```python
from build123d import *

# Parameters (mm, degrees)
BOSS_EXTRUDE1_DEPTH = 513.461
SKETCH2_R           = 19.05
CUT_EXTRUDE1_DEPTH  = 31.75
SKETCH3_R           = 3.2258
CUT_EXTRUDE2_DEPTH  = 31.75
SKETCH4_R           = 11.500000003
CUT_EXTRUDE3_DEPTH  = 499.872


with BuildPart() as part:
    # Sketch1 → Boss-Extrude1 (new body)
    with BuildSketch(Plane.XY):
        with BuildLine():
            Line((-159.385, 0), (-158.115, 0))
            ThreePointArc((-158.115, 0), (-154.073884746, -1.673884746), (-152.4, -5.715))
            Line((-152.4, -5.715), (-152.4, -16.91))
            ThreePointArc((-152.4, -16.91), (-150.726115254, -20.951115254), (-146.685, -22.625))
            Line((-146.685, -22.625), (-125.96, -22.625))
            ThreePointArc((-125.96, -22.625), (-121.918884746, -24.298884746), (-120.245, -28.34))
            Line((-120.245, -28.34), (-120.245, -57.40750012))
            ThreePointArc((-120.245, -57.40750012), (-118.571115254, -61.448615374), (-114.53, -63.12250012))
            Line((-114.53, -63.12250012), (-107.315, -63.12250012))
            ThreePointArc((-107.315, -63.12250012), (-103.273884746, -61.448615374), (-101.6, -57.40750012))
            Line((-101.6, -57.40750012), (-101.6, 0))
            Line((-101.6, 0), (-101.6, 38.17350945))
            ThreePointArc((-101.6, 38.17350945), (-99.926115254, 42.214624704), (-95.885, 43.88850945))
            Line((-95.885, 43.88850945), (95.885, 43.88850945))
            ThreePointArc((95.885, 43.88850945), (99.926115254, 42.214624704), (101.6, 38.17350945))
            Line((101.6, 38.17350945), (101.6, 0))
            Line((101.6, 0), (101.6, -57.40750012))
            ThreePointArc((101.6, -57.40750012), (103.273884746, -61.448615374), (107.315, -63.12250012))
            Line((107.315, -63.12250012), (114.53, -63.12250012))
            ThreePointArc((114.53, -63.12250012), (118.571115254, -61.448615374), (120.245, -57.40750012))
            Line((120.245, -57.40750012), (120.245, -28.34))
            ThreePointArc((120.245, -28.34), (121.918884746, -24.298884746), (125.96, -22.625))
            Line((125.96, -22.625), (146.685, -22.625))
            ThreePointArc((146.685, -22.625), (150.726115254, -20.951115254), (152.4, -16.91))
            Line((152.4, -16.91), (152.4, -5.715))
            ThreePointArc((152.4, -5.715), (154.073884746, -1.673884746), (158.115, 0))
            Line((158.115, 0), (159.385, 0))
            ThreePointArc((159.385, 0), (163.426115254, 1.673884746), (165.1, 5.715))
            Line((165.1, 5.715), (165.1, 59.52))
            ThreePointArc((165.1, 59.52), (157.660512242, 77.480512242), (139.7, 84.92))
            Line((139.7, 84.92), (-139.7, 84.92))
            ThreePointArc((-139.7, 84.92), (-157.660512242, 77.480512242), (-165.1, 59.52))
            Line((-165.1, 59.52), (-165.1, 5.715))
            ThreePointArc((-165.1, 5.715), (-163.426115254, 1.673884746), (-159.385, 0))
        make_face()
    extrude(amount=BOSS_EXTRUDE1_DEPTH)

    # Sketch2 → Cut-Extrude1 (cut)
    with BuildSketch(Plane(origin=(0, 84.92, 0), x_dir=(1, 0, 0), z_dir=(0, 1, 0))):
        with Locations(Location((-50.8, -25.4, 0), (0, 0, 270))):
            Circle(SKETCH2_R)
        with Locations(Location((50.8, -25.4, 0), (0, 0, 270))):
            Circle(SKETCH2_R)
        with Locations(Location((50.8, -488.061, 0), (0, 0, 270))):
            Circle(SKETCH2_R)
        with Locations(Location((-50.8, -488.061, 0), (0, 0, 270))):
            Circle(SKETCH2_R)
    extrude(amount=-CUT_EXTRUDE1_DEPTH, mode=Mode.SUBTRACT)

    # Sketch3 → Cut-Extrude2 (cut)
    with BuildSketch(Plane(origin=(0, 53.17, 0), x_dir=(1, 0, 0), z_dir=(0, 1, 0))):
        with Locations(Location((-50.8, -25.4, 0), (0, 0, 270))):
            Circle(SKETCH3_R)
        with Locations(Location((50.8, -25.4, 0), (0, 0, 270))):
            Circle(SKETCH3_R)
        with Locations(Location((50.8, -488.061, 0), (0, 0, 270))):
            Circle(SKETCH3_R)
        with Locations(Location((-50.8, -488.061, 0), (0, 0, 270))):
            Circle(SKETCH3_R)
    extrude(amount=-CUT_EXTRUDE2_DEPTH, mode=Mode.SUBTRACT)

    # Sketch4 → Cut-Extrude3 (cut)
    with BuildSketch(Plane.ZY.offset(165.1)):
        with Locations(Location((344.866041788, 12.13850945, 0), (0, 0, 326.043312317))):
            Circle(SKETCH4_R)
        with Locations(Location((197.228541788, 12.13850945, 0), (0, 0, 326.043312317))):
            Circle(SKETCH4_R)
    extrude(amount=-CUT_EXTRUDE3_DEPTH, mode=Mode.SUBTRACT)


solid = part.part
```
Could you check a few things on this model? Use its own coordinates, in mm. A direction names the side the tool comes from. Coordinates: 2 decimals unless noted, no trailing zeros. Loops run counter-clockwise (first coordinate to the right, second up) from the corner with the lowest first, then second, coordinate; pieces in that order, holes last. Notation, with made-up numbers: M 72,-30 L 82,-30 A25 cw 82,6 Z; hole C 11,-11 d11. An arc over 180 degrees is marked long. Put each result on its own line as item: value. Start each with the question number.
(1) Thinking about a two-plate mould opening in Y: for faces 5 (the face through (132.906, 11.432, 333.388)), 6 (the face through (-51, 53.17, 29)), 7 (the face through (-49.96, 69.27, 469.03)), which applies, pulls with the +Y half, pulls with the -Y half, needs draft (parallel to the pull), parting line crosses it, or undercut?
(2) Suppose I cut it at C-C on x = -75. Please give me the cut outline in (y, z), then the cut area to 3 significant figures.
(3) Suppose I cut it at D-D on y = 68.5. Please give me the cut outline in (x, z), then the cut area to 3 significant figures.
(4) Suppose I cut it at A-A on y = 30. Please give me the cut outline in (x, z), then the cut area to 3 significant figures.
(5) For faces 1 (the face through (-120.245, -43, 253)), 2 (the face through (-1, 43.889, 253)), 3 (the face through (120.245, -43, 253)), 4 (the face through (-31.912, 69.267, 22.92)), which set-ups out of +Z, -Z, +X, -X, +Y, -Y let a thin tool reach every point of the face, with its end or its side?
(6) I need wall thicknesses on line 1 (X direction, y = 47, z = 25.4); line 2 (Z direction, x = 50, y = 72); line 3 (X direction, y = -27.5, z = 387.5). Which ranges of each line are inside material? Lowest first, please. Write a range as from..to.
(7) Will these pins go through, and if not, where does the flat tip stop? P1, Ø1.5, axis at x = 113.5, y = 23.5, coming from the -Z side; P2, Ø11.5, axis at x = 59, z = 494.5, coming from the +Y side; P3, Ø10.5, axis at x = 137, z = 203.5, coming from the -Y side (3 decimals); P4, Ø5.5, axis at y = -13.5, z = 281.5, coming from the -X side.
Solutions:
1. face 5: undercut
1. face 6: pulls with the +Y half
1. face 7: needs draft
2. outline: M 43.89,0 L 84.92,0 L 84.92,513.46 L 43.89,513.46 Z
2. area: 21,100 mm2
3. outline: M -163.46,0 L 163.46,0 L 163.46,513.46 L -163.46,513.46 Z; hole C -50.8,25.4 d38.1; hole C -50.8,488.06 d38.1; hole C 50.8,25.4 d38.1; hole C 50.8,488.06 d38.1
3. area: 163,000 mm2
4. outline: M -165.1,0 L -101.6,0 L -101.6,513.46 L -165.1,513.46 Z; M 101.6,0 L 165.1,0 L 165.1,513.46 L 101.6,513.46 Z
4. area: 65,200 mm2
5. face 1: +Z, -Z, -X, -Y
5. face 2: +Z, -Z, -Y
5. face 3: +Z, -Z, +X, -Y
5. face 4: +Y
6. line 1: x = -165.1..-54.03, -47.57..47.57, 54.03..165.1
6. line 2: z = 0..6.37, 44.43..469.03, 507.09..513.46
6. line 3: x = -120.31..-101.6, 101.6..120.31
7. P1: stops at z = 0
7. P2: stops at y = 53.17
7. P3: stops at y = -22.625
7. P4: stops at x = -152.4
